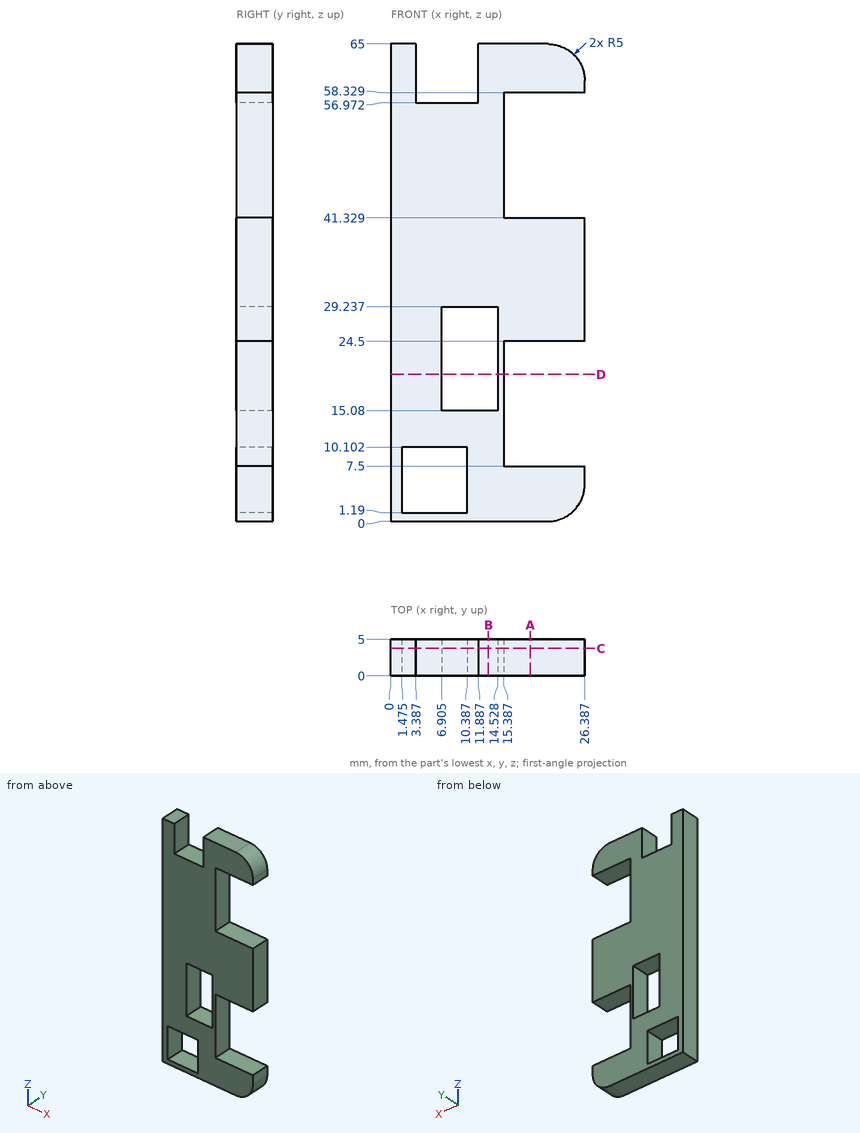
Print and shaded views of the part. All mm, measured from the part's lowest x, y and z. Round coordinates to 2 decimals unless told otherwise and drop trailing zeros. Write each loop counter-clockwise with the first axis right and the second up, starting at its lowest first coordinate (ties: lowest second). Pieces come first, ordered by that corner, then holes. Notation, with made-up numbers: (26, 19) -> (65, 19) arc R13 cw to (65, 30) -> close; hole circle Ø10 at (68.25, -7.5). An arc over 180 degrees is marked (long way). Return JSON: item names as keys, results as strings. Group by question number.
Q1. Saw through at A-A on x = 19. Write the cut outline in (y, z).
Q2. Saw through at B-B on x = 13.25. Write the cut outline in (y, z), plus the area to 3 significant figures.
Q3. Pin check, flat tips, straight feed: pin 1 (1.5 mm diameter, centred on x = 10.5, y = 2, fed in from +Z); pin 2 (2.5 mm diameter, centred on y = 3, z = 61.5, fed in from +X); pin 3 (1.5 mm diameter, centred on y = 3, z = 49.5, fed in from +X). Stop position of each tip, or through.
Q4. Saw through at C-C on y = 3.75. Write the cut outline in (x, z) (1 decimal), plus the area to 4 significant figures.
Q5. Probe L1, parallel to Z at x = 7, y = 4.05; L2, parallel to Z at x = 18, y = 4.3; L3, parallel to X at y = 1.55, z = 10 (1 decimal). List the from-to ranges inside material, lowest first. Write a range as [from, to].
Q6. Saw through at D-D on z = 20. Write the cut outline in (x, y) (1 decimal).
Answer:
{
 "1": {"outline": "(0, 0) -> (5, 0) -> (5, 7.5) -> (0, 7.5) -> close; (0, 24.5) -> (5, 24.5) -> (5, 41.33) -> (0, 41.33) -> close; (0, 58.33) -> (5, 58.33) -> (5, 65) -> (0, 65) -> close"},
 "2": {"outline": "(0, 0) -> (5, 0) -> (5, 15.08) -> (0, 15.08) -> close; (0, 29.24) -> (5, 29.24) -> (5, 65) -> (0, 65) -> close", "area": "254 mm2"},
 "3": {"pin 1": "z = 56.97", "pin 2": "x = 26.38", "pin 3": "x = 15.39"},
 "4": {"outline": "(0, 0) -> (21.4, 0) arc R5 ccw to (26.4, 5) -> (26.4, 7.5) -> (15.4, 7.5) -> (15.4, 24.5) -> (26.4, 24.5) -> (26.4, 41.3) -> (15.4, 41.3) -> (15.4, 58.3) -> (26.4, 58.3) -> (26.4, 60) arc R5 ccw to (21.4, 65) -> (11.9, 65) -> (11.9, 57) -> (3.4, 57) -> (3.4, 65) -> (0, 65) -> close; hole (1.5, 1.2) -> (10.4, 1.2) -> (10.4, 10.1) -> (1.5, 10.1) -> close; hole (6.9, 15.1) -> (14.5, 15.1) -> (14.5, 29.2) -> (6.9, 29.2) -> close", "area": "1,075 mm2"},
 "5": {"L1": "[0, 1.19], [10.1, 15.08], [29.24, 56.97]", "L2": "[0, 7.5], [24.5, 41.33], [58.33, 65]", "L3": "[0, 1.5], [10.4, 15.4]"},
 "6": {"outline": "(0, 0) -> (6.9, 0) -> (6.9, 5) -> (0, 5) -> close; (14.5, 0) -> (15.4, 0) -> (15.4, 5) -> (14.5, 5) -> close"}
}
